```python
from build123d import *

# Parameters (mm, degrees)
F0_W     = 304.8
F0_H     = 76.2
F1_DEPTH = 25.4
F2_W     = 304.8
F2_H     = 25.4
F3_DEPTH = 50.8
F4_R     = 12.5
F5_DEPTH = 25.4
F6_SIZE  = 12


with BuildPart() as f1:
    # F0 (on Top) → F1 (new body)
    with BuildSketch(Plane.XY):
        Rectangle(F0_W, F0_H)
    extrude(amount=F1_DEPTH)

    # F2 (on face) → F3 (join)
    with BuildSketch(Plane.XY.offset(25.4)):
        Rectangle(F2_W, F2_H)
    extrude(amount=F3_DEPTH)

    # F4 (on face) → F5 (join)
    with BuildSketch(Plane(origin=(0, 0, 0), x_dir=(1, 0, 0), z_dir=(0, 0, -1))):
        with Locations((-76.2, 0)):
            Circle(F4_R)
        with Locations((76.2, 0)):
            Circle(F4_R)
    extrude(amount=F5_DEPTH)

    # F6
    f6_edges = [f1.edges().sort_by_distance(p)[0] for p in [
        (-88.7, 0, -25.4),
        (63.7, 0, -25.4),
    ]]
    chamfer(f6_edges, length=F6_SIZE)


solid = f1.part
```
Check sheet for the modelled part. Datum: model origin and axes. Units: mm. A direction names the side the tool comes from. Coordinates: 2 decimals unless noted, no trailing zeros. Order: outer loops, then holes, each group sorted by start corner. A loop starts at its lowest first (then second) coordinate and runs counter-clockwise, first axis right, second up. Notation, with made-up numbers: (56.5, 22.25) -> (82.5, 22.25) arc R25 cw to (82.5, 54.25) -> close; hole circle Ø6 at (-25, 79.5). An arc over 180 degrees is marked (long way). Write each question's results on one line, items separated by ' | '. Start each with the question number.
1) Section check B-B (y = 24.5). Enter the section's corners in (x, z), and give its area (3 significant figures).
2) Material ranges on line 1 along Y through (x, z) = (73, 40); line 2 along Z through (x, y) = (51, -28.5); line 3 along Z through (x, y) = (124, 4.5), recorded low to high.
3) Draft check along X on faces 1 (the face through (-2, 12.7, 50)), 2 (the face through (152.4, -1, 29)), 3 (the face through (63.712, -0.55, -6.606)). Enter one of: pulls with the +X half, pulls with the -X half, needs draft (parallel to the pull), parting line crosses it, or undercut.
4) Section check A-A (x = 0.5). Enter the section's corners in (y, z), and give its area (3 significant figures).
5) Set-up check for faces 4 (the face through (-2, 38.1, 13)), 5 (the face through (-64.277, -3.755, -6.606)), 6 (the face through (-2, -25, 25.4)), 7 (the face through (-2, 26, 25.4)): record each of +Z, -Z, +X, -X, +Y, -Y from which the full face is reachable in a straight line by a thin tool's end or side.
6) Depth check by flat-ended pin: pin 1 (3 mm diameter, centred on x = -112, y = 7.5, fed in from -Z); pin 2 (2 mm diameter, centred on x = 52, z = 51.5, fed in from -Y); pin 3 (3 mm diameter, centred on x = 100, z = 39, fed in from +Y). Enter the tip coordinate at first touch or a pass-through.
7) Section check C-C (z = 47.5). Enter the section's corners in (x, y), and give its area (3 significant figures).
Checked values:
1) outline: (-152.4, 0) -> (152.4, 0) -> (152.4, 25.4) -> (-152.4, 25.4) -> close | area: 7,740 mm²
2) line 1: -12.7 to 12.7 | line 2: 0 to 25.4 | line 3: 0 to 76.2
3) face 1: needs draft | face 2: pulls with the +X half | face 3: undercut
4) outline: (-38.1, 0) -> (38.1, 0) -> (38.1, 25.4) -> (12.7, 25.4) -> (12.7, 76.2) -> (-12.7, 76.2) -> (-12.7, 25.4) -> (-38.1, 25.4) -> close | area: 3,230 mm²
5) face 4: +Z, -Z, +X, -X, +Y | face 5: -Z | face 6: +Z, +X, -X, -Y | face 7: +Z, +X, -X, +Y
6) pin 1: z = 0 | pin 2: y = -12.7 | pin 3: y = 12.7
7) outline: (-152.4, -12.7) -> (152.4, -12.7) -> (152.4, 12.7) -> (-152.4, 12.7) -> close | area: 7,740 mm²
